```python
from build123d import *


with BuildPart() as f1:
    # F0 (on Front) → F1 (revolve)
    with BuildSketch(Plane.XZ):
        Polygon((5, 12.5), (0, 7.5), (2.5, 7.5), (7.5, 12.5), align=None)
        Polygon((0, 7.5), (0, 5), (2.5, 5), (2.5, 6.25), (2.5, 7.5), align=None)
        Polygon((2.5, 5), (0, 5), (5, 0), (7.5, 0), align=None)
    revolve(axis=Axis((12.5, 0, 9.325136), (0, 0, 1)))


solid = f1.part
```
Geometry: final body of the model. Coordinates: model frame, mm. A direction names the side the tool comes from. Round coordinates to 2 decimals unless told otherwise and drop trailing zeros. Order: outer loops, then holes, each group sorted by start corner. A loop starts at its lowest first (then second) coordinate and runs counter-clockwise, first axis right, second up. Notation, with made-up numbers: (-18, 10.25) -> (16, 10.25) arc R18 ccw to (16, 33.25) -> close; hole circle Ø3 at (27.5, 70.25). An arc over 180 degrees is marked (long way). Use CSV: the item, a comma, the result in double quotes. Start each with the question number.
1) Material intervals for line 1 along Y through (x, z) = (12.5, 6.5); line 2 along X through (y, z) = (0, 5.9); line 3 along Z through (x, y) = (8, -6.75), sorted ascending. Write a range as from..to.
2) Draft query along Y for faces 3 (the face through (14, 5, 12.5)), 4 (the face through (7.433, -1.596, 0.313)), 5 (the face through (21.71, -8.45, 6.23)). Return one class per face: +Y half, -Y half, draft (parallel to the pull), parting line (faces both ways), or undercut.
3) Section D-D (z = 2.5). Return the cut outline in (x, y), and give its area (3 significant figures).
4) Set-up query: faces 1 (the face through (20.235, -0.34, 0.243)), 2 (the face through (2.96, -3, 6.27)). Return all of +Z, -Z, +X, -X, +Y, -Y with unobstructed straight access to the full face (end or side cutting, diameter ignored); none if empty.
5) First-contact query: pin 1 Ø5 at (x, z) = (17.5, 8.5) entering from -Y; pin 2 Ø1 at (y, z) = (-9, 9.5) entering from -X; pin 3 Ø3 at (x, z) = (18.5, 11) entering from +Y. Flat tips, straight axial feed; report the tip coordinate or a pass-through.
6) Section B-B (y = 0). Return the cut outline in (x, z).
7) Section A-A (x = 12.5). Return the cut outline in (y, z).
8) Section C-C (z = 6.75). Return the cut outline in (x, y), and give its area (3 significant figures).
Returned:
1,line 1,"y = -12.5..-10, 10..12.5"
1,line 2,"x = 0..2.5, 22.5..25"
1,line 3,"z = 0.61..3.11, 9.39..11.89"
2,face 3,"draft"
2,face 4,"undercut"
2,face 5,"parting line"
3,outline,"circle Ø20 at (12.5, 0); hole circle Ø15 at (12.5, 0)"
3,area,"137 mm²"
4,face 1,"-Z"
4,face 2,"none"
5,pin 1,"stops at y = -12.2"
5,pin 2,"stops at x = 5.93"
5,pin 3,"stops at y = 8.86"
6,outline,"(0, 5) -> (5, 0) -> (7.5, 0) -> (2.5, 5) -> (2.5, 7.5) -> (7.5, 12.5) -> (5, 12.5) -> (0, 7.5) -> close; (17.5, 0) -> (20, 0) -> (25, 5) -> (25, 7.5) -> (20, 12.5) -> (17.5, 12.5) -> (22.5, 7.5) -> (22.5, 5) -> close"
7,outline,"(-12.5, 5) -> (-7.5, 0) -> (-5, 0) -> (-10, 5) -> (-10, 7.5) -> (-5, 12.5) -> (-7.5, 12.5) -> (-12.5, 7.5) -> close; (5, 0) -> (7.5, 0) -> (12.5, 5) -> (12.5, 7.5) -> (7.5, 12.5) -> (5, 12.5) -> (10, 7.5) -> (10, 5) -> close"
8,outline,"circle Ø25 at (12.5, 0); hole circle Ø20 at (12.5, 0)"
8,area,"177 mm²"
